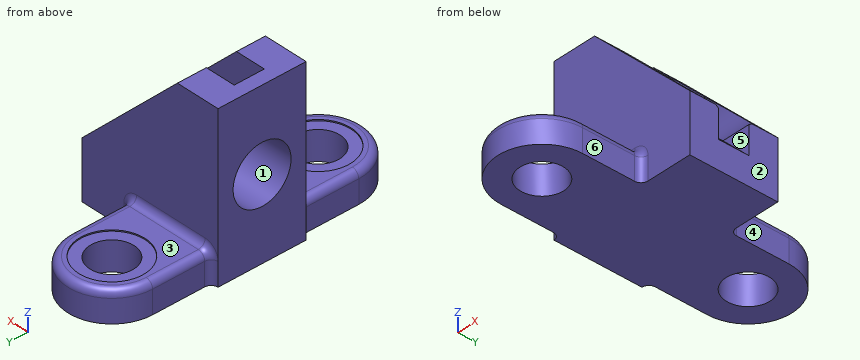
```python
from build123d import *

# Parameters (mm, degrees)
F1_DEPTH  = 38
F3_DEPTH  = 13
F5_DEPTH  = 26
F6_R      = 19
F7_DEPTH  = 26.001
F6_R_2    = 28.5
F8_DEPTH  = 1
F9_R      = 5.99999
F11_R     = 25
F12_DEPTH = 127.001


# Not quite as in the source:
# - a fillet or chamfer is up to 0.001 mm smaller than in the source, because OpenCascade refuses the exact size


with BuildPart() as f1:
    # F0 (on Front) → F1 (new body)
    with BuildSketch(Plane.XZ):
        Polygon((-60.1392750332, 139), (-60.1392750332, 0), (66.8607249668, 0), (66.8607249668, 50), (-22.1392750332, 139), align=None)
    extrude(amount=F1_DEPTH)

    # F2 (on face) → F3 (cut)
    with BuildSketch(Plane(origin=(0, 0, 0), x_dir=(-1, 0, 0), z_dir=(0, 1, 0))):
        Polygon((-66.8607249668, 24), (48.1392750332, 139), (22.1392750332, 139), (-66.8607249668, 50), align=None)
    extrude(amount=-F3_DEPTH, mode=Mode.SUBTRACT)

    # F4 (on Top) → F5 (join)
    with BuildSketch(Plane.XY):
        with BuildLine():
            Line((21.8607249668, -38), (-54.1392750332, -38))
            Line((-54.1392750332, -38), (-54.1392750332, -89))
            ThreePointArc((-54.1392750332, -89), (-16.1392750332, -127), (21.8607249668, -89))
            Line((21.8607249668, -89), (21.8607249668, -38))
        make_face()
    extrude(amount=F5_DEPTH)

    # F6 (on face) → F7 (cut, through all)
    with BuildSketch(Plane.XY.offset(26)):
        with Locations((-16.1392750332, -89)):
            Circle(F6_R)
    extrude(amount=-F7_DEPTH, mode=Mode.SUBTRACT)

    # F6 (on face) → F8 (cut)
    with BuildSketch(Plane.XY.offset(26)):
        with Locations((-16.1392750332, -89)):
            Circle(F6_R_2)
        with Locations((-16.1392750332, -89)):
            Circle(F6_R, mode=Mode.SUBTRACT)
    extrude(amount=-F8_DEPTH, mode=Mode.SUBTRACT)

    # F9 (radius 6 in the source; OpenCascade refuses exactly that, so slightly less here)
    f9_edges = [f1.edges().sort_by_distance(p)[0] for p in [
        (-16.139275, -38, 26),
        (21.860725, -38, 13),
        (-54.139275, -38, 13),
        (-54.139275, -63.5, 26),
    ]]
    fillet(f9_edges, radius=F9_R)

    # F10: F1 across plane


with BuildPart() as f1_1:
    add(f1.part)
    add(f1.part.mirror(Plane.XZ))

    # F11 (on face) → F12 (cut, through all)
    with BuildSketch(Plane(origin=(-60.1392750332, 0, 0), x_dir=(0, -1, 0), z_dir=(-1, 0, 0))):
        with Locations((0, 69.5)):
            Circle(F11_R)
    extrude(amount=-F12_DEPTH, mode=Mode.SUBTRACT)


solid = f1_1.part
```
Geometry: final body of the model. Coordinates: model frame, mm. Face numbers are marked on the shaded views. A direction names the side the tool comes from. Coordinates: 2 decimals unless noted, no trailing zeros. Order: outer loops, then holes, each group sorted by start corner. A loop starts at its lowest first (then second) coordinate and runs counter-clockwise, first axis right, second up.
Item 1: Section query B-B (y = 0). Output: boundary loops of the cut face in (x, z), then the cut area to 3 significant figures.
Answer:
outline: (-60.14, 0) - (66.86, 0) - (66.86, 24) - (46.36, 44.5) - (-60.14, 44.5) - close; (-60.14, 94.5) - (-3.64, 94.5) - (-48.14, 139) - (-60.14, 139) - close
area: 6,970 mm2
Item 2: Draft query along Z for the marked faces 1, 2 and 3. Return one class per face: released by +Z, released by -Z, zero draft, split by the parting line, or undercut.
Answer:
face 1: undercut
face 2: zero draft
face 3: released by +Z
Item 3: Material intervals for line 1 along Y through (x, z) = (-25, 11); line 2 along Z through (x, y) = (1, -66.5); line 3 along X through (y, z) = (99.5, 6.5), sorted ascending.
Answer:
line 1: y = -125.95 to -105.81, -72.19 to 72.19, 105.81 to 125.95
line 2: z = 0 to 25
line 3: x = -52.66 to -31.97, -0.3 to 20.38
Item 4: Contact query for flat-ended pins moving along their axis: P1, Ø6, axis at x = 19.5, y = -57, coming from the +Z side; P2, Ø8, axis at x = 32.5, z = 49, coming from the +Y side; P3, Ø16, axis at y = -55.5, z = 7.5, coming from the -X side. Output: stop coordinate, or through.
Answer:
P1: stops at z = 25.97
P2: stops at y = 38
P3: stops at x = -54.14
Item 5: Section query D-D (y = 28.5). Output: boundary loops of the cut face in (x, z), then the cut area to 3 significant figures.
Answer:
outline: (-60.14, 0) - (66.86, 0) - (66.86, 50) - (-22.14, 139) - (-60.14, 139) - close
area: 13,700 mm2
Item 6: Section query A-A (z = 69.5). Output: boundary loops of the cut face in (x, y).
Answer:
outline: (-60.14, -38) - (47.36, -38) - (47.36, -25) - (-60.14, -25) - close; (-60.14, 25) - (47.36, 25) - (47.36, 38) - (-60.14, 38) - close
Item 7: Access query for the marked faces 4, 5 and 6. Directions: +Z, -Z, +X, -X, +Y, -Y. A direction counts if a zero-diameter tool reaches every point of the face in a straight line with its end or side. Return the directions, or none.
Answer:
face 4: +Z, -Z, +X, +Y
face 5: +Z, +X
face 6: +Z, -Z, +X, -Y
Item 8: Section query C-C (x = -29). State how many separate pieces and enclosed holes the cut face has, then the cut area to 3 significant figures.
Answer:
separate pieces: 3
enclosed holes: 1
area: 11,100 mm2
